Part model, mm, in its own coordinate system. Face numbers are marked on the shaded views. A direction names the side the tool comes from. Round coordinates to 2 decimals unless told otherwise and drop trailing zeros. Write each loop counter-clockwise with the first axis right and the second up, starting at its lowest first coordinate (ties: lowest second). Pieces come first, ordered by that corner, then holes.
1) Saw through at B-B on x = 5. Write the cut outline in (y, z), and give its area (3 significant figures).
2) Which spindle directions (+Z, -Z, +X, -X, +Y, -Y) get a long thin tool onto all of the face, cutting with end or side? Do the marked faces 1, 2, 3, 4 and 5. Say none if no direction does.
3) Saw through at C-C on x = 1.75. Write the cut outline in (y, z), and give its area (3 significant figures).
4) Saw through at A-A on y = 4.25. Write the cut outline in (x, z), and give its area (3 significant figures).
5) Drill centre lines: L1, parallel to Y at x = 2, z = -0.7; L2, parallel to X at y = 4.25, z = 1.45; L3, parallel to X at y = -4, z = 0.35. Where is each one in solid material? Low to high.
6) Pull direction X, two halves, no side cores. Call the marked faces 6, 7 and 8: +X half, -X half, draft (parallel to the pull), parting line (faces both ways), or undercut.
7) Flat gauge pin, fed straight in: pin 1 (1.5 mm diameter, centred on y = 2, z = -0.5, fed in from -X). Where does the tip first touch, or does it go through?
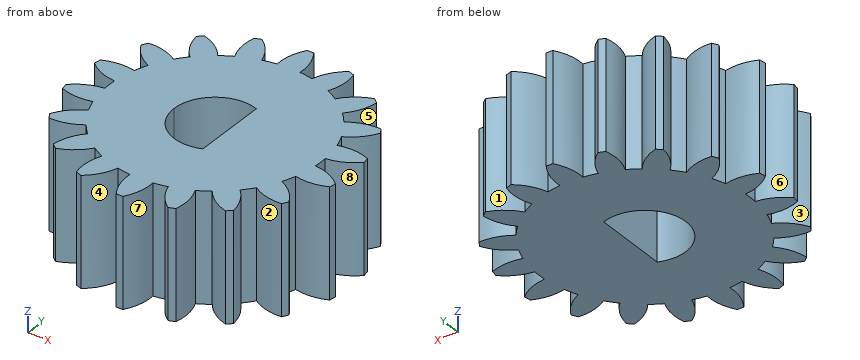
```python
from build123d import *

# Parameters (mm, degrees)
BASPROSKE_W           = 4
BASPROSKE_H           = 5
TOOTHCUT_DEPTH        = 9.124038405
TEETHCUTS_COUNT       = 18
TEETHCUTS_ANGLE       = 340
BORE_DEPTH            = 50.0000508
BODY_MOVE_COPY1_ANGLE = 90
BODY_MOVE_COPY2_ANGLE = 90


with BuildPart() as part:
    # BasProSke → Base-Revolve (revolve)
    with BuildSketch(Plane(origin=(0, 0, 0), x_dir=(1, 0, 0), z_dir=(0, 1, 0)), mode=Mode.PRIVATE) as base_revolve_sk:
        with Locations((2, 2.5)):
            Rectangle(BASPROSKE_W, BASPROSKE_H)
    revolve(base_revolve_sk.sketch.rotate(Axis((-10, 0, 0), (1, 0, 0)), 180), axis=Axis((-10, 0, 0), (1, 0, 0)))

    # TooCutSke → ToothCut (cut, through all)
    with BuildSketch(Plane(origin=(0, 0, 0), x_dir=(0, 0, -1), z_dir=(1, 0, 0))):
        with BuildLine():
            ThreePointArc((0.25527463, 3.865580275), (0, 3.874), (-0.25527463, 3.865580275))
            ThreePointArc((-0.25527463, 3.865580275), (-0.416281865, 4.46052923), (-0.768562654, 4.96628197))
            ThreePointArc((-0.768562654, 4.96628197), (0, 5.0254), (0.768562654, 4.96628197))
            ThreePointArc((0.768562654, 4.96628197), (0.416281865, 4.46052923), (0.25527463, 3.865580275))
        make_face()
    toothcut = extrude(amount=TOOTHCUT_DEPTH, mode=Mode.SUBTRACT)

    # TeethCuts: ToothCut ×18 about axis
    teethcuts_axis = Axis((-10, 0, 0), (1, 0, 0))
    for i in range(1, TEETHCUTS_COUNT):
        add(toothcut.rotate(teethcuts_axis, i * TEETHCUTS_ANGLE / (TEETHCUTS_COUNT - 1)), mode=Mode.SUBTRACT)

    # BorSke → Bore (cut, symmetric)
    with BuildSketch(Plane(origin=(0, 0, 0), x_dir=(0, 0, -1), z_dir=(1, 0, 0))):
        with BuildLine():
            ThreePointArc((-1.401240549, 0.535280228), (-1.235499968, -0.850611444), (0, -1.5))
            Line((0, -1.5), (0, 0.535280228))
            Line((0, 0.535280228), (-1.401240549, 0.535280228))
        make_face()
        with BuildLine():
            Line((0, 0.535280228), (0, -1.5))
            ThreePointArc((0, -1.5), (1.060660172, -1.060660172), (1.5, 0))
            ThreePointArc((1.5, 0), (1.475103526, 0.272157285), (1.401240549, 0.535280228))
            Line((1.401240549, 0.535280228), (0, 0.535280228))
        make_face()
    extrude(amount=BORE_DEPTH, both=True, mode=Mode.SUBTRACT)


with BuildPart() as part_1:
    # Body-Move/Copy1: moved
    add(part.part.rotate(Axis((2, 0, 0), (0, 0, -1)), BODY_MOVE_COPY1_ANGLE))


with BuildPart() as part_2:
    # Body-Move/Copy2: moved
    add(part_1.part.rotate(Axis((0, 0, 0), (1, 0, 0)), BODY_MOVE_COPY2_ANGLE))


solid = part_2.part
```
Completed:
1. outline: (-3.87, -2) - (-2.93, -2) - (-2.93, 2) - (-3.87, 2) - close; (-2.45, -2) - (2.45, -2) - (2.45, 2) - (-2.45, 2) - close; (2.93, -2) - (3.87, -2) - (3.87, 2) - (2.93, 2) - close
1. area: 27.2 mm2
2. face 1: +Z, -Z, +Y
2. face 2: +Z, -Z
2. face 3: +Z, -Z, -X
2. face 4: +Z, -Z, -Y
2. face 5: +Z, -Z, +X
3. outline: (-4.78, -2) - (-1.48, -2) - (-1.48, 2) - (-4.78, 2) - close; (1.48, -2) - (4.78, -2) - (4.78, 2) - (1.48, 2) - close
3. area: 26.4 mm2
4. outline: (0.12, -2) - (0.86, -2) - (0.86, 2) - (0.12, 2) - close; (1.59, -2) - (2.41, -2) - (2.41, 2) - (1.59, 2) - close; (3.14, -2) - (3.88, -2) - (3.88, 2) - (3.14, 2) - close
4. area: 9.18 mm2
5. L1: y = -5 to -1.5, 1.5 to 5
5. L2: x = 0.12 to 0.86, 1.59 to 2.41, 3.14 to 3.88
5. L3: x = 0.14 to 0.99, 1.57 to 2.43, 3.01 to 3.86
6. face 6: -X half
6. face 7: undercut
6. face 8: +X half
7. pin 1: stops at x = -2.39
